from build123d import *

# Parameters (mm, degrees)
F1_DEPTH = 75
F2_W     = 25
F2_H     = 24
F2_H_2   = 26.113208
F3_DEPTH = 20
F4_W     = 25
F4_H     = 24
F5_DEPTH = 20


with BuildPart() as f1:
    # F0 (on Front) → F1 (new body)
    with BuildSketch(Plane.XZ):
        Polygon((-30, 0), (0, 0), (0, 72), (-20, 72), (-20, 19.773584), (-90, 19.773584), (-90, 72), (-110, 72), (-110, 0), (-80, 0), (-80, 12), (-30, 12), align=None)
    extrude(amount=F1_DEPTH)

    # F2 (on face) → F3 (cut)
    with BuildSketch(Plane.YZ.offset(-90)):
        with Locations((-62.5, 60)):
            Rectangle(F2_W, F2_H)
        with Locations((-12.5, 58.943396)):
            Rectangle(F2_W, F2_H_2)
    extrude(amount=-F3_DEPTH, mode=Mode.SUBTRACT)

    # F4 (on face) → F5 (cut)
    with BuildSketch(Plane(origin=(-20, 0, 0), x_dir=(0, -1, 0), z_dir=(-1, 0, 0))):
        with Locations((37.5, 60)):
            Rectangle(F4_W, F4_H)
    extrude(amount=-F5_DEPTH, mode=Mode.SUBTRACT)


solid = f1.part
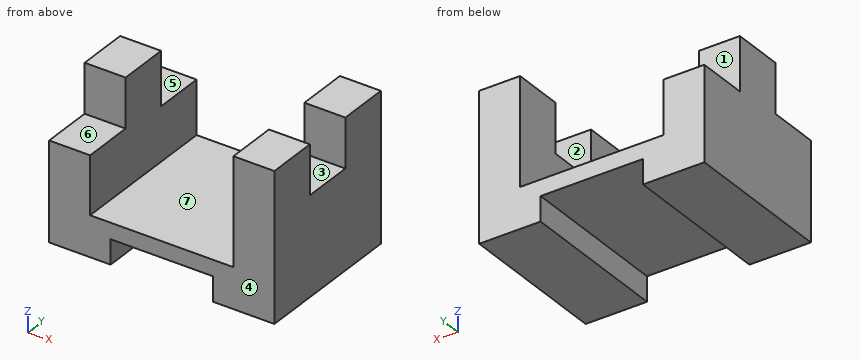
Input: part model. Units: mm. Frame: model coordinates. Face numbers are marked on the shaded views. A direction names the side the tool comes from. Give positions to 0.01 mm unless a question says otherwise; leave off trailing zeros. Loops run counter-clockwise (first coordinate to the right, second up) from the corner with the lowest first, then second, coordinate; pieces in that order, holes last. Notation, with made-up numbers: M 76,49.25 L 109,49.25 A10 ccw 109,58.25 Z; hole C 46,17 d11. An arc over 180 degrees is marked long. Use CSV: the item, a comma, the result in double quotes.
(1) Set-up query: the marked faces 5, 6 and 7. Return all of +Z, -Z, +X, -X, +Y, -Y with unobstructed straight access to the full face (end or side cutting, diameter ignored); none if empty.
Outcome:
face 5,"+Z, -X, +Y"
face 6,"+Z, -X, -Y"
face 7,"+Z, +Y, -Y"
(2) Pull-direction query (Y, two-part tool) for the marked faces 1, 2, 3 and 4; classes: pulls with the +Y half, pulls with the -Y half, needs draft (parallel to the pull), parting line crosses it, or undercut.
Outcome:
face 1,"pulls with the +Y half"
face 2,"undercut"
face 3,"undercut"
face 4,"pulls with the -Y half"
(3) Section D-D, the plane z = 54. Return loops of the section in (x, y), plus the area to 3 significant figures.
Outcome:
outline,"M -110,-50 L -90,-50 L -90,-25 L -110,-25 Z; M -20,-75 L 0,-75 L 0,-50 L -20,-50 Z; M -20,-25 L 0,-25 L 0,0 L -20,0 Z"
area,"1,500 mm²"
(4) Section C-C, the plane y = -60. Return loops of the section in (x, z).
Outcome:
outline,"M -110,0 L -80,0 L -80,12 L -30,12 L -30,0 L 0,0 L 0,72 L -20,72 L -20,19.77 L -90,19.77 L -90,48 L -110,48 Z"
(5) Section B-B, the plane x = -14.5. Return loops of the section in (y, z).
Outcome:
outline,"M -75,0 L 0,0 L 0,72 L -25,72 L -25,48 L -50,48 L -50,72 L -75,72 Z"
(6) Material intervals for L1, parallel to X at y = -29.5, z = 24.5; L2, parallel to X at y = -6, z = 66; L3, parallel to X at y = -60, z = 7.5, sorted ascending. Write a range as [from, to].
Outcome:
L1,"x = [-110, -90], [-20, 0]"
L2,"x = [-20, 0]"
L3,"x = [-110, -80], [-30, 0]"
(7) Pin query (flat end, axial travel): P1, Ø10, axis at x = -101.5, y = -12.5, coming from the +Z side; P2, Ø1, axis at y = -32.5, z = 64.5, coming from the +X side; P3, Ø10, axis at x = -96, z = 54.5, coming from the +Y side. Return the tip coordinate at first contact, or that it passes through.
Outcome:
P1,"stops at z = 45.89"
P2,"stops at x = -90"
P3,"stops at y = -25"
(8) Section A-A, the plane z = 41.5. Return loops of the section in (x, y).
Outcome:
outline,"M -110,-75 L -90,-75 L -90,0 L -110,0 Z; M -20,-75 L 0,-75 L 0,0 L -20,0 Z"
